Geometry check sheet. Reference: the model listing, model coordinates, mm. A direction names the side the tool comes from. Give positions to 0.01 mm unless a question says otherwise; leave off trailing zeros. Write each loop counter-clockwise with the first axis right and the second up, starting at its lowest first coordinate (ties: lowest second). Pieces come first, ordered by that corner, then holes. Notation, with made-up numbers: (69, 43) -> (82, 43) arc R31 ccw to (82, 77) -> close; hole circle Ø8 at (-13.75, 10.25). An arc over 180 degrees is marked (long way). Write item = value, one per line. Start each with the question number.
1. Cross-section at B-B, the plane z = -50. Record the cut outline in (x, y), plus the area to 3 significant figures.
2. Set-up check for faces 1 (the flat face through (18, 7, -60.291)), 2 (the flat face through (10.929, 7, -28)): record each of +Z, -Z, +X, -X, +Y, -Y from which the full face is reachable in a straight line by a thin tool's end or side.
3. Cross-section at A-A, the plane y = 8.5. Record the cut outline in (x, z), plus the area to 3 significant figures.
4. Thickness scan on line 1 along X through (y, z) = (2.75, -0.5); line 2 along Z through (x, y) = (11.5, 1); line 3 along X through (y, z) = (7.5, 24). Record the ranges inside material, lowest first.
5. Cross-section at C-C, the plane x = 3.25. Record the cut outline in (y, z).
6. Mould release check, pull along X, two halves, no side actions. Record for faces 3 (the flat face through (13, 0, -11)), 4 (the cylindrical face through (17.714, 7.605, 11.365)), 5 (the cylindrical face through (2.925, 7.605, 37.604)): pulls with the +X half, pulls with the -X half, needs draft (parallel to the pull), parting line crosses it, or undercut.
7. Depth check by flat-ended pin: P1, Ø3, axis at x = 15.93, z = 11.6, coming from the +Y side; P2, Ø4, axis at x = 10.5, y = 13, coming from the -Z side; P3, Ø1.5, axis at x = 4.5, y = 9.5, coming from the +Z side; P4, Ø4.5, axis at y = 4.5, z = -15, coming from the -X side. Enter the tip coordinate at first touch or a pass-through.
```python
from build123d import *

# Parameters (mm, degrees)
BOSS_EXTRUDE1_DEPTH = 15
FILLET1_R           = 7
SKETCH2_R           = 1.8
CUT_EXTRUDE1_DEPTH  = 66.559736532
FILLET3_R           = 7
FILLET5_R           = 7
CHAMFER2_SIZE       = 5


with BuildPart() as part:
    # Sketch1 → Boss-Extrude1 (new body)
    with BuildSketch(Plane(origin=(0, 0, 0), x_dir=(1, 0, 0), z_dir=(0, 1, 0))):
        Polygon((10.928961749, 60.29143898), (10.928961749, 0.29143898), (0.928961749, -29.70856102), (0.928961749, -39.70856102), (10.928961749, -39.70856102), (20.928961749, -9.70856102), (20.928961749, 60.29143898), align=None)
    extrude(amount=BOSS_EXTRUDE1_DEPTH)

    # Fillet1
    fillet1_edges = [part.edges().sort_by_distance(p)[0] for p in [
        (0.928961749, 7.5, 39.70856102),
    ]]
    fillet(fillet1_edges, radius=FILLET1_R)

    # Sketch2 → Cut-Extrude1 (cut, through all)
    with BuildSketch(Plane(origin=(0, 15, 0), x_dir=(1, 0, 0), z_dir=(0, 1, 0))):
        with Locations(Location((15.928961749, -11.599196317, 0), (0, 0, 270))):
            Circle(SKETCH2_R)
        with Locations(Location((7.928961749, -32.70856102, 0), (0, 0, 270))):
            Circle(SKETCH2_R)
    extrude(amount=-CUT_EXTRUDE1_DEPTH, mode=Mode.SUBTRACT)

    # Fillet3
    # the kernel refuses this fillet: 7 mm, written as the material it takes off along each edge
    with BuildSketch(Plane(origin=(10.928961749, -11.713900217, 39.70856102), x_dir=(-1, 0, 0), z_dir=(0, 1, 0))) as fillet3_piece_1:
        with BuildLine():
            CenterArc((5.159078888, -6.658706958), FILLET3_R, 107.965233202, 53.599817975)
            Line((-1.481704199, -4.445112596), (-1.61451986, -4.400840709))
            Line((-1.61451986, -4.400840709), (-0.132815662, 0.044271887))
            Line((-0.132815662, 0.044271887), (0, 0.14))
            ThreePointArc((0, 0.14), (1.5, 0.14), (2.956818422, 0.133174139))
            Line((2.956818422, 0.133174139), (3, 0))
        make_face()
    extrude(amount=38.427800433, mode=Mode.SUBTRACT)

    # Fillet5
    fillet5_edges = [part.edges().sort_by_distance(p)[0] for p in [
        (20.928961749, 7.5, 9.70856102),
    ]]
    fillet(fillet5_edges, radius=FILLET5_R)

    # Chamfer2
    chamfer2_edges = [part.edges().sort_by_distance(p)[0] for p in [
        (10.928961749, 7.5, -60.29143898),
    ]]
    chamfer(chamfer2_edges, length=CHAMFER2_SIZE)


solid = part.part
```
Answers:
q1.outline = (10.93, 0) -> (20.93, 0) -> (20.93, 15) -> (10.93, 15) -> close
q1.area = 150 mm^2
q2.face_1 = -Z, +X, -X, +Y, -Y
q2.face_2 = -Z, -X, +Y, -Y
q3.outline = (0.93, 29.71) -> (10.93, -0.29) -> (10.93, -55.29) -> (15.93, -60.29) -> (20.93, -60.29) -> (20.93, 8.57) arc R7 ccw to (20.57, 10.79) -> (12.41, 35.26) arc R7 ccw to (7.93, 39.71) arc R7 ccw to (0.93, 32.71) -> close; hole circle Ø3.6 at (7.93, 32.71); hole circle Ø3.6 at (15.93, 11.6)
q3.area = 1,050 mm^2
q4.line_1 = 10.93 to 20.93
q4.line_2 = -55.86 to 37.07
q4.line_3 = 2.83 to 16.17
q5.outline = (0, 22.75) -> (15, 22.75) -> (15, 37.92) -> (0, 37.92) -> close
q6.face_3 = needs draft
q6.face_4 = undercut
q6.face_5 = pulls with the -X half
q7.P1 = through
q7.P2 = -56.86
q7.P3 = 39.18
q7.P4 = 10.93
